Part model, mm, in its own coordinate system. Coordinates: 2 decimals unless noted, no trailing zeros. Loops run counter-clockwise (first coordinate to the right, second up) from the corner with the lowest first, then second, coordinate; pieces in that order, holes last. Notation, with made-up numbers: M -20,52.5 L 29,52.5 A27 cw 29,88.5 Z; hole C 16.5,-40 d5. An arc over 180 degrees is marked long. Answer as a JSON object with one key per item and string values. Group by question number.
1. Saw through at A-A on z = 3.35. Write the cut outline in (x, y), then the cut area to 3 significant figures.
2. Drop flat-ended pins along their axis: pin 1 Ø0.6 at (y, z) = (9.5, 3) entering from +X; pin 2 Ø1.1 at (x, z) = (-10.5, 3.5) entering from +Y; pin 3 Ø0.6 at (y, z) = (13.5, 3) entering from -X. Give the stop position or say it passes through.
3. Saw through at D-D on x = 12. Write the cut outline in (y, z).
4. Saw through at B-B on y = 7. Write the cut outline in (x, z), then the cut area to 3 significant figures.
5. Saw through at C-C on x = 5. Write the cut outline in (y, z), then the cut area to 3 significant figures.
6. Drill centre lines: L1, parallel to Z at x = 1.5, y = 1.5; L2, parallel to X at y = 8.5, z = 3.45; L3, parallel to Y at x = -8, z = 2.8. Where is each one in solid material? Low to high.
from build123d import *

# Parameters (mm, degrees)
F1_DEPTH = 4.318
F0_W     = 37.719
F0_H     = 27.559
F2_DEPTH = 2.159
F3_SIZE  = 1.0795


with BuildPart() as f1:
    # F0 (on Top) → F1 (new body)
    with BuildSketch(Plane.XY):
        Polygon((-11.915093, 11.556174), (-16.995093, 16.636174), (-16.995093, 11.556174), align=None)
        Polygon((-11.915093, 11.556174), (-16.995093, 11.556174), (-16.995093, 6.476174), align=None)
        Polygon((-11.915093, 6.476174), (-11.915093, 11.556174), (-16.995093, 6.476174), align=None)
        Polygon((-11.915093, 6.476174), (-16.995093, 6.476174), (-11.915093, 1.396174), align=None)
        Polygon((-6.835093, 16.636174), (-11.915093, 16.636174), (-6.835093, 11.556174), align=None)
        Polygon((-1.755093, 11.556174), (-6.835093, 16.636174), (-6.835093, 11.556174), align=None)
        Polygon((-1.755093, 16.636174), (-6.835093, 16.636174), (-1.755093, 11.556174), align=None)
        Polygon((3.324907, 11.556174), (-1.755093, 16.636174), (-1.755093, 11.556174), align=None)
        Polygon((3.324907, 11.556174), (-1.755093, 11.556174), (-1.755093, 6.476174), (3.324907, 1.396174), (8.404907, 1.396174), (3.324907, 6.476174), align=None)
        Polygon((-6.835093, 6.476174), (-11.915093, 6.476174), (-11.915093, 1.396174), (-1.755093, 1.396174), align=None)
    extrude(amount=F1_DEPTH)

    # F0 (on Top) → F2 (join)
    with BuildSketch(Plane.XY):
        with Locations((-4.295093, 9.016174)):
            Rectangle(F0_W, F0_H)
        Polygon((-16.995093, 11.556174), (-16.995093, 16.636174), (-11.915093, 11.556174), (-11.915093, 6.476174), (-6.835093, 6.476174), (-1.755093, 1.396174), (-11.915093, 1.396174), (-16.995093, 6.476174), align=None, mode=Mode.SUBTRACT)
        Polygon((-6.835093, 11.556174), (-11.915093, 16.636174), (-6.835093, 16.636174), (-1.755093, 16.636174), (3.324907, 11.556174), (3.324907, 6.476174), (8.404907, 1.396174), (3.324907, 1.396174), (-1.755093, 6.476174), (-1.755093, 11.556174), align=None, mode=Mode.SUBTRACT)
    extrude(amount=F2_DEPTH)

    # F3
    f3_edges = [f1.edges().sort_by_distance(p)[0] for p in [
        (-4.295093, 22.795674, 2.159),
        (-23.154593, 9.016174, 2.159),
        (14.564407, 9.016174, 2.159),
        (-4.295093, -4.763326, 2.159),
    ]]
    chamfer(f3_edges, length=F3_SIZE)


solid = f1.part
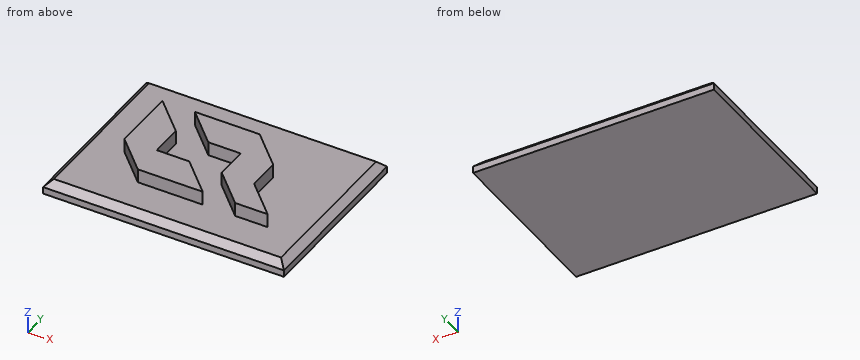
Outcome:
{
 "1": {"outline": "M -17,6.48 L -11.92,1.4 L -1.76,1.4 L -6.84,6.48 L -11.92,6.48 L -11.92,11.56 L -17,16.64 Z; M -11.92,16.64 L -6.84,11.56 L -1.76,11.56 L -1.76,6.48 L 3.32,1.4 L 8.4,1.4 L 3.32,6.48 L 3.32,11.56 L -1.76,16.64 Z", "area": "194 mm²"},
 "2": {"pin 1": "stops at x = 3.32", "pin 2": "stops at y = 16.64", "pin 3": "stops at x = -17"},
 "3": {"outline": "M -4.76,0 L 22.8,0 L 22.8,1.08 L 21.72,2.16 L -3.68,2.16 L -4.76,1.08 Z"},
 "4": {"outline": "M -23.15,0 L 14.56,0 L 14.56,1.08 L 13.48,2.16 L 3.32,2.16 L 3.32,4.32 L -1.76,4.32 L -1.76,2.16 L -11.92,2.16 L -11.92,4.32 L -17,4.32 L -17,2.16 L -22.08,2.16 L -23.15,1.08 Z", "area": "102 mm²"},
 "5": {"outline": "M -4.76,0 L 22.8,0 L 22.8,1.08 L 21.72,2.16 L 4.8,2.16 L 4.8,4.32 L 1.4,4.32 L 1.4,2.16 L -3.68,2.16 L -4.76,1.08 Z", "area": "65.7 mm²"},
 "6": {"L1": "z = 0 to 2.16", "L2": "x = -17 to -11.92, -1.76 to 3.32", "L3": "y = 1.4 to 6.48, 12.72 to 16.64"}
}
